Geometry: final body of the model. Coordinates: model frame, mm. Face numbers are marked on the shaded views. Give positions to 0.01 mm unless a question says otherwise; leave off trailing zeros. Order: outer loops, then holes, each group sorted by start corner. A loop starts at its lowest first (then second) coordinate and runs counter-clockwise, first axis right, second up. Notation, with made-up numbers: (30, -3.5) - (86, -3.5) arc R4 cw to (86, 2.5) - close; hole circle Ø9 at (-38.75, 78.5). An arc over 180 degrees is marked (long way). Put each result on its own line as item: value. Start each with the question number.
1. Section B-B on y = 0. Return the cut outline in (x, z).
2. Section C-C on z = 2. Return the cut outline in (x, y), plus the area to 3 significant figures.
3. Section D-D on y = 10. Return the cut outline in (x, z), plus the area to 3 significant figures.
4. Ray query, line 1 along Y through (x, z) = (0, 8.25); line 2 along Y through (x, z) = (0, 5.25); line 3 along Y through (x, z) = (3.5, 4.5). Return the intervals inside material, ascending. Write a range as from..to.
5. Mould query, pull axis Y, two halves, no side actions, for the marked faces 1, 2, 3 and 4. Classes: pulls with the +Y half, pulls with the -Y half, needs draft (parallel to the pull), parting line crosses it, or undercut.
6. Section A-A on x = 0. Return the cut outline in (y, z), plus the area to 3 significant figures.
7. First-contact query: P1, Ø1.6, axis at x = 0, y = 16.5, coming from the +Z side. Flat tip, straight axial feed; report the tip coordinate or a pass-through.
from build123d import *

# Parameters (mm, degrees)
BOX003_W                    = 25
BOX003_H                    = 5
BOX003_DEPTH                = 6
CYLINDER_R                  = 7.6
CYLINDER_DEPTH              = 10
CYLINDER004_R               = 1.65
CYLINDER004_DEPTH           = 9
CYLINDER005_R               = 1.65
CYLINDER005_DEPTH           = 9
BOX_W                       = 4
BOX_H                       = 68
BOX_DEPTH                   = 4
BOX002_W                    = 4
BOX002_H                    = 68
BOX002_DEPTH                = 4
CYLINDER003_W               = 28
CYLINDER003_H               = 10
CYLINDER003_ANGLE           = 26
CYLINDER003_PLACEMENT_ANGLE = 103
CYLINDER002_W               = 32
CYLINDER002_H               = 10
CYLINDER002_ANGLE           = 26
CYLINDER002_PLACEMENT_ANGLE = 103
BOX001_W                    = 25
BOX001_H                    = 68
BOX001_DEPTH                = 10


with BuildPart() as obj1:
    # Box003 → Box003 (new body)
    with BuildSketch(Plane(origin=(-12.5, 33, 0), x_dir=(1, 0, 0), z_dir=(0, 0, 1))):
        with Locations((12.5, 2.5)):
            Rectangle(BOX003_W, BOX003_H)
    extrude(amount=BOX003_DEPTH)


with BuildPart() as zylinder:
    # Cylinder → Cylinder (new body)
    with BuildSketch(Plane.XY):
        Circle(CYLINDER_R)
    extrude(amount=CYLINDER_DEPTH)


with BuildPart() as zylinder003:
    # Cylinder004 → Cylinder004 (new body)
    with BuildSketch(Plane(origin=(0, -12, 1), x_dir=(1, 0, 0), z_dir=(0, 0, 1))):
        Circle(CYLINDER004_R)
    extrude(amount=CYLINDER004_DEPTH)


with BuildPart() as zylinder004:
    # Cylinder005 → Cylinder005 (new body)
    with BuildSketch(Plane(origin=(0, 16, 1), x_dir=(1, 0, 0), z_dir=(0, 0, 1))):
        Circle(CYLINDER005_R)
    extrude(amount=CYLINDER005_DEPTH)


with BuildPart() as obj2:
    # Box → Box (new body)
    with BuildSketch(Plane(origin=(8.5, -35, 6), x_dir=(1, 0, 0), z_dir=(0, 0, 1))):
        with Locations((2, 34)):
            Rectangle(BOX_W, BOX_H)
    extrude(amount=BOX_DEPTH)


with BuildPart() as obj3:
    # Box002 → Box002 (new body)
    with BuildSketch(Plane(origin=(-12.5, -35, 6), x_dir=(1, 0, 0), z_dir=(0, 0, 1))):
        with Locations((2, 34)):
            Rectangle(BOX002_W, BOX002_H)
    extrude(amount=BOX002_DEPTH)


with BuildPart() as zylinder002:
    # Cylinder003 → Cylinder003 (revolve)
    with BuildSketch(Plane.XZ):
        with Locations((14, 5)):
            Rectangle(CYLINDER003_W, CYLINDER003_H)
    revolve(axis=Axis((0, 0, 0), (0, 0, 1)), revolution_arc=CYLINDER003_ANGLE)


with BuildPart() as zylinder002_1:
    # Cylinder003 placement: moved
    add(zylinder002.part.rotate(Axis((0, 0, 0), (0, 0, -1)), CYLINDER003_PLACEMENT_ANGLE))


with BuildPart() as fusion:
    # Cylinder002 → Cylinder002 (revolve)
    with BuildSketch(Plane.XZ):
        with Locations((16, 5)):
            Rectangle(CYLINDER002_W, CYLINDER002_H)
    revolve(axis=Axis((0, 0, 0), (0, 0, 1)), revolution_arc=CYLINDER002_ANGLE)


with BuildPart() as fusion_1:
    # Cylinder002 placement: moved
    add(fusion.part.rotate(Axis((0, 0, 0), (0, 0, -1)), CYLINDER002_PLACEMENT_ANGLE))

    # Cut001: cut Zylinder002
    add(zylinder002_1.part, mode=Mode.SUBTRACT)

    # Fusion: union Zylinder, Zylinder003, Zylinder004, obj2, obj3
    add(zylinder.part)
    add(zylinder003.part)
    add(zylinder004.part)
    add(obj2.part)
    add(obj3.part)


with BuildPart() as fusion001:
    # Box001 → Box001 (new body)
    with BuildSketch(Plane(origin=(-12.5, -35, 0), x_dir=(1, 0, 0), z_dir=(0, 0, 1))):
        with Locations((12.5, 34)):
            Rectangle(BOX001_W, BOX001_H)
    extrude(amount=BOX001_DEPTH)

    # Cut: cut Fusion
    add(fusion_1.part, mode=Mode.SUBTRACT)

    # Fusion001: union obj1
    add(obj1.part)


solid = fusion001.part
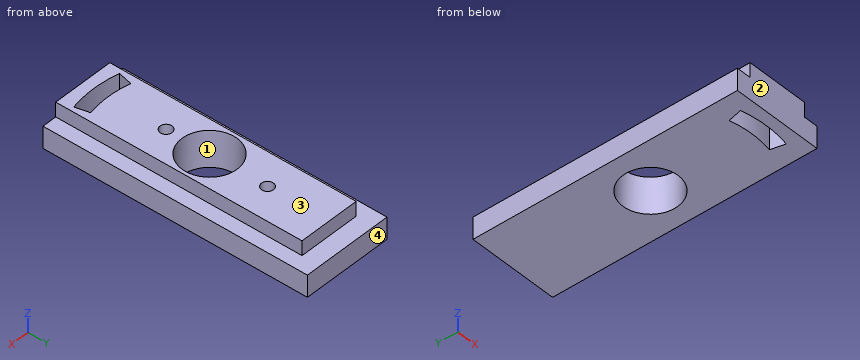
Resolved:
1. outline: (-12.5, 0) - (-7.6, 0) - (-7.6, 10) - (-8.5, 10) - (-8.5, 6) - (-12.5, 6) - close; (7.6, 0) - (12.5, 0) - (12.5, 6) - (8.5, 6) - (8.5, 10) - (7.6, 10) - close
2. outline: (-12.5, -35) - (12.5, -35) - (12.5, 38) - (-12.5, 38) - close; hole circle Ø15.2 at (0, 0); hole (-7.2, -31.18) arc R32 ccw to (7.2, -31.18) - (6.3, -27.28) arc R28 cw to (-6.3, -27.28) - close; hole circle Ø3.3 at (0, -12); hole circle Ø3.3 at (0, 16)
2. area: 1,570 mm^2
3. outline: (-12.5, 0) - (12.5, 0) - (12.5, 6) - (8.5, 6) - (8.5, 10) - (-8.5, 10) - (-8.5, 6) - (-12.5, 6) - close
3. area: 218 mm^2
4. line 1: -35..-32, -28..-13.65, -10.35..-7.6, 7.6..14.35, 17.65..33
4. line 2: -35..-32, -28..-13.65, -10.35..-7.6, 7.6..14.35, 17.65..38
4. line 3: -35..-31.81, -27.78..-6.75, 6.75..38
5. face 1: undercut
5. face 2: pulls with the -Y half
5. face 3: needs draft
5. face 4: pulls with the +Y half
6. outline: (-35, 0) - (-32, 0) - (-32, 10) - (-35, 10) - close; (-28, 0) - (-7.6, 0) - (-7.6, 10) - (-10.35, 10) - (-10.35, 1) - (-13.65, 1) - (-13.65, 10) - (-28, 10) - close; (7.6, 0) - (38, 0) - (38, 6) - (33, 6) - (33, 10) - (17.65, 10) - (17.65, 1) - (14.35, 1) - (14.35, 10) - (7.6, 10) - close
6. area: 459 mm^2
7. P1: z = 1
